Autodesk Inventor part; units mm, degrees
ref_plane "YZ Plane" through (0, 0, 0) normal (1, 0, 0) x (0, 1, 0)
ref_plane "XZ Plane" through (0, 0, 0) normal (0, 1, 0) x (-1, 0, 0)
ref_plane "XY Plane" through (0, 0, 0) normal (0, 0, 1) x (1, 0, 0)
sketch "スケッチ1" plane through (0, 0, 0) normal (0, 0, 1) x (1, 0, 0)
  arc A0 (-3.88, 6.4184) -> (-3.2378, 4.1327) centre (2.5862, 7.0023) ccw
  arc A1 (-3.2378, 4.1327) -> (-3.7123, 3.7123) centre (0, 0) ccw
  arc A2 (-3.7123, 3.7123) -> (-5.9039, 4.6254) centre (-7.263, -1.7233) ccw
  arc A3 (-5.9039, 4.6254) -> (-6.4184, 3.88) centre (0, 0) ccw
  arc A4 (-6.4184, 3.88) -> (-4.7875, 2.1547) centre (-0.9641, 7.4021) ccw
  arc A5 (-4.7875, 2.1547) -> (-5.0123, 1.5619) centre (0, 0) ccw
  arc A6 (-5.0123, 1.5619) -> (-7.3771, 1.3519) centre (-5.6302, -4.9012) ccw
  arc A7 (-7.3771, 1.3519) -> (-7.4863, 0.4528) centre (0, 0) ccw
  arc A8 (-7.4863, 0.4528) -> (-5.2404, -0.317) centre (-4.2936, 6.1062) ccw
  arc A9 (-5.2404, -0.317) -> (-5.164, -0.9463) centre (0, 0) ccw
  arc A10 (-5.164, -0.9463) -> (-7.1604, -2.2313) centre (-2.7076, -6.9563) ccw
  arc A11 (-7.1604, -2.2313) -> (-6.8392, -3.0781) centre (0, 0) ccw
  arc A12 (-6.8392, -3.0781) -> (-4.4929, -2.716) centre (-6.6395, 3.4114) ccw
  arc A13 (-4.4929, -2.716) -> (-4.1327, -3.2378) centre (0, 0) ccw
  arc A14 (-4.1327, -3.2378) -> (-5.3033, -5.3033) centre (0.8353, -7.4178) ccw
  arc A15 (-5.3033, -5.3033) -> (-4.6254, -5.9039) centre (0, 0) ccw
  arc A16 (-4.6254, -5.9039) -> (-2.716, -4.4929) centre (-7.4644, -0.0649) ccw
  arc A17 (-2.716, -4.4929) -> (-2.1547, -4.7875) centre (0, 0) ccw
  arc A18 (-2.1547, -4.7875) -> (-2.2313, -7.1604) centre (4.1868, -6.1799) ccw
  arc A19 (-2.2313, -7.1604) -> (-1.3519, -7.3771) centre (0, 0) ccw
  arc A20 (-1.3519, -7.3771) -> (-0.317, -5.2404) centre (-6.5792, -3.5263) ccw
  arc A21 (-0.317, -5.2404) -> (0.317, -5.2404) centre (0, 0) ccw
  arc A22 (0.317, -5.2404) -> (1.3519, -7.3771) centre (6.5792, -3.5263) ccw
  arc A23 (1.3519, -7.3771) -> (2.2313, -7.1604) centre (0, 0) ccw
  arc A24 (2.2313, -7.1604) -> (2.1547, -4.7875) centre (-4.1868, -6.1799) ccw
  arc A25 (2.1547, -4.7875) -> (2.716, -4.4929) centre (0, 0) ccw
  arc A26 (2.716, -4.4929) -> (4.6254, -5.9039) centre (7.4644, -0.0649) ccw
  arc A27 (4.6254, -5.9039) -> (5.3033, -5.3033) centre (0, 0) ccw
  arc A28 (5.3033, -5.3033) -> (4.1327, -3.2378) centre (-0.8353, -7.4178) ccw
  arc A29 (4.1327, -3.2378) -> (4.4929, -2.716) centre (0, 0) ccw
  arc A30 (4.4929, -2.716) -> (6.8392, -3.0781) centre (6.6395, 3.4114) ccw
  arc A31 (6.8392, -3.0781) -> (7.1604, -2.2313) centre (0, 0) ccw
  arc A32 (7.1604, -2.2313) -> (5.164, -0.9463) centre (2.7076, -6.9563) ccw
  arc A33 (5.164, -0.9463) -> (5.2404, -0.317) centre (0, 0) ccw
  arc A34 (5.2404, -0.317) -> (7.4863, 0.4528) centre (4.2936, 6.1062) ccw
  arc A35 (7.4863, 0.4528) -> (7.3771, 1.3519) centre (0, 0) ccw
  arc A36 (7.3771, 1.3519) -> (5.0123, 1.5619) centre (5.6302, -4.9012) ccw
  arc A37 (5.0123, 1.5619) -> (4.7875, 2.1547) centre (0, 0) ccw
  arc A38 (4.7875, 2.1547) -> (6.4184, 3.88) centre (0.9641, 7.4021) ccw
  arc A39 (6.4184, 3.88) -> (5.9039, 4.6254) centre (0, 0) ccw
  arc A40 (5.9039, 4.6254) -> (3.7123, 3.7123) centre (7.263, -1.7233) ccw
  arc A41 (3.7123, 3.7123) -> (3.2378, 4.1327) centre (0, 0) ccw
  arc A42 (3.2378, 4.1327) -> (3.88, 6.4184) centre (-2.5862, 7.0023) ccw
  arc A43 (3.88, 6.4184) -> (3.0781, 6.8392) centre (0, 0) ccw
  arc A44 (3.0781, 6.8392) -> (1.5619, 5.0123) centre (7.2319, 1.8493) ccw
  arc A45 (1.5619, 5.0123) -> (0.9463, 5.164) centre (0, 0) ccw
  arc A46 (0.9463, 5.164) -> (0.4528, 7.4863) centre (-5.5441, 4.9983) ccw
  arc A47 (0.4528, 7.4863) -> (-0.4528, 7.4863) centre (0, 0) ccw
  arc A48 (-0.4528, 7.4863) -> (-0.9463, 5.164) centre (5.5441, 4.9983) ccw
  arc A49 (-0.9463, 5.164) -> (-1.5619, 5.0123) centre (0, 0) ccw
  arc A50 (-1.5619, 5.0123) -> (-3.0781, 6.8392) centre (-7.2319, 1.8493) ccw
  arc A51 (-3.0781, 6.8392) -> (-3.88, 6.4184) centre (0, 0) ccw
sketch "スケッチ2" plane through (0, 0, 0) normal (0, 0, 1) x (1, 0, 0)
  line L0 (-2, 1.5) -> (2, 1.5)
  line L1 (2, -1.5) -> (-2, -1.5)
  arc A0 (-2, 1.5) -> (-2, -1.5) centre (0, 0) ccw
  arc A1 (2, -1.5) -> (2, 1.5) centre (0, 0) ccw
  point P0 (0, 0)
  point P1 (0, 0)
  point P2 (0, 0)
  point P3 (0, 0)
  point P4 (0, 0)
  point P5 (0, 0)
  point P6 (0, 0)
  point P7 (0, 0)
  point P8 (0, 0)
  point P9 (0, 0)
  point P10 (0, 0)
  point P11 (0, 0)
  point P12 (0, 0)
  point P13 (0, 0)
  point P14 (0, 0)
  point P15 (0, 0)
  point P16 (0, 0)
  point P17 (0, 0)
  point P18 (0, 0)
  point P19 (0, 0)
  point P20 (0, 0)
  point P21 (0, 0)
  point P22 (0, 0)
  point P23 (0, 0)
  point P24 (0, 0)
  point P25 (0, 0)
extrude "押し出し1" add sketch "スケッチ1" along normal blind 6.5
extrude "押し出し2" cut sketch "スケッチ2" along normal blind 6.5
properties part number "Gear13"
The listing builds one solid part. Answer for the finished solid, in the listing's coordinates (mm). A direction names the side the tool comes from. Coordinates: 2 decimals unless noted, no trailing zeros. Order: outer loops, then holes, each group sorted by start corner. A loop starts at its lowest first (then second) coordinate and runs counter-clockwise, first axis right, second up. Notation, with made-up numbers: M -27,-5 L 20,-5 A21 cw 20,20 Z; hole C 66.5,-23 d5. An arc over 180 degrees is marked long. Answer as a JSON object with one key per item and string values. Group by question number.
1. Section B-B on y = 2.5 is taken. Write down the section's boundary in (x, z), then the cut area to 3 significant figures.
2. Determine the mould class of faces 6 (the cylindrical face through (3.619, -5.296, 3.204)), 7 (the cylindrical face through (-7.446, 0.898, 3.204)), 8 (the cylindrical face through (6.21, -1.49, 3.2)) for opening direction Y: released by +Y, released by -Y, zero draft, split by the parting line, or undercut.
3. Section C-C on y = -2.5 is taken. Write down the section's boundary in (x, z), then the cut area to 3 significant figures.
4. Section A-A on x = 3.5 is taken. Write down the section's boundary in (y, z), then the cut area to 3 significant figures.
5. Straight lines are drawn through the part: line 1 (Y direction, x = -0.25, z = 3); line 2 (X direction, y = 4, z = 0.5); line 3 (Y direction, x = -5.5, z = 2). For each, find the intervals that lie inside material, in ascending order.
6. A tool of negligible diameter and unlimited length cuts with its end or side. For faces 1 (the cylindrical face through (-5.633, -3.003, 3.204)), 2 (the cylindrical face through (-2.25, 6.01, 3.2)), 3 (the cylindrical face through (-0.73, -6.34, 3.2)), 4 (the cylindrical face through (-6.38, -0.04, 3.2)), 5 (the cylindrical face through (6.41, -0.03, 3.2)), from which of +Z, -Z, +X, -X, +Y, -Y can it reach the whole face along a straight path? Write none if from no direction.
7. Flat-ended cylindrical pins translate along their axes: P1, Ø1, axis at y = -3, z = 4, coming from the -X side; P2, Ø1.2, axis at x = 1, z = 2.5, coming from the +Y side; P3, Ø2, axis at y = -4, z = 2, coming from the +X side. Find the tip coordinate at first contact, or state that the pin passes through.
Values follow:
{
 "1": {"outline": "M -5.22,0 L 5.22,0 L 5.22,6.5 L -5.22,6.5 Z", "area": "67.9 mm2"},
 "2": {"face 6": "released by -Y", "face 7": "released by +Y", "face 8": "undercut"},
 "3": {"outline": "M -7.07,0 L 7.07,0 L 7.07,6.5 L -7.07,6.5 Z", "area": "91.9 mm2"},
 "4": {"outline": "M -5.21,0 L 3.91,0 L 3.91,6.5 L -5.21,6.5 Z; M 4.74,0 L 6.63,0 L 6.63,6.5 L 4.74,6.5 Z", "area": "71.6 mm2"},
 "5": {"line 1": "-5.24 to -1.5, 1.5 to 7.5", "line 2": "-6.34 to -4.2, -3.4 to 3.4, 4.2 to 6.34", "line 3": "-2.98 to -1.09, -0.27 to 1.59, 2.76 to 4.53"},
 "6": {"face 1": "+Z, -Z", "face 2": "+Z, -Z, +Y", "face 3": "+Z, -Z, -Y", "face 4": "+Z, -Z, -X", "face 5": "+Z, -Z, +X"},
 "7": {"P1": "x = -7.07", "P2": "y = 7.49", "P3": "x = 6.87"}
}
